from build123d import *

# Parameters (mm, degrees)
BOSS_EXTRUDE1_DEPTH    = 2
BOSS_EXTRUDE1_2_DEPTH  = 2
BOSS_EXTRUDE1_3_DEPTH  = 2
BOSS_EXTRUDE1_4_DEPTH  = 2
BOSS_EXTRUDE1_5_DEPTH  = 2
BOSS_EXTRUDE1_6_DEPTH  = 2
BOSS_EXTRUDE1_7_DEPTH  = 2
BOSS_EXTRUDE1_8_DEPTH  = 2
BOSS_EXTRUDE1_9_DEPTH  = 2
BOSS_EXTRUDE1_10_DEPTH = 2
SKETCH3_R              = 30
SKETCH3_R_2            = 16.5
BOSS_EXTRUDE2_DEPTH    = 2
SKETCH4_R              = 2.9
BOSS_EXTRUDE3_DEPTH    = 2
SKETCH6_R              = 5
BOSS_EXTRUDE4_DEPTH    = 1
SKETCH13_R             = 4.177329345
BOSS_EXTRUDE6_DEPTH    = 2
FILLET2_R              = 0.5
SKETCH14_R             = 3
CUT_EXTRUDE1_DEPTH     = 20


with BuildPart() as part:
    # Sketch2 → Boss-Extrude1 (new body)
    with BuildSketch(Plane.XY.offset(10)):
        with BuildLine():
            Line((8.357492916, 13.704694326), (1.290071734, 3.973134201))
            Line((1.290071734, 3.973134201), (1.290510646, 1.776982243))
            Line((1.290510646, 1.776982243), (3.379039645, 2.45604795))
            Line((3.379039645, 2.45604795), (10.446460828, 12.187608075))
            ThreePointArc((10.446460828, 12.187608075), (10.160519997, 13.990635156), (8.357492916, 13.704694326))
        make_face()
    extrude(amount=BOSS_EXTRUDE1_DEPTH)


with BuildPart() as body_2:
    # Sketch2 → Boss-Extrude1 2 (new body)
    with BuildSketch(Plane.XY.offset(10)):
        with BuildLine():
            Line((1.290071734, 3.973134201), (1.287668054, 16.000257666))
            ThreePointArc((1.287668054, 16.000257666), (-0.003455665, 17.290865413), (-1.294063412, 15.999741695))
            Line((-1.294063412, 15.999741695), (-1.291659732, 3.972618229))
            Line((-1.291659732, 3.972618229), (-0.000438912, 2.196151958))
            Line((-0.000438912, 2.196151958), (1.290071734, 3.973134201))
        make_face()
    extrude(amount=BOSS_EXTRUDE1_2_DEPTH)


with BuildPart() as body_3:
    # Sketch2 → Boss-Extrude1 3 (new body)
    with BuildSketch(Plane.XY.offset(10)):
        with BuildLine():
            Line((-1.29122082, 1.776466271), (-1.291659732, 3.972618229))
            Line((-1.291659732, 3.972618229), (-8.362970151, 13.701352658))
            ThreePointArc((-8.362970151, 13.701352658), (-10.166111381, 13.986572778), (-10.451331501, 12.183431547))
            Line((-10.451331501, 12.183431547), (-3.380021082, 2.454697118))
            Line((-3.380021082, 2.454697118), (-1.29122082, 1.776466271))
        make_face()
    extrude(amount=BOSS_EXTRUDE1_3_DEPTH)


with BuildPart() as body_4:
    # Sketch2 → Boss-Extrude1 4 (new body)
    with BuildSketch(Plane.XY.offset(10)):
        with BuildLine():
            Line((-2.088800262, 0.678230847), (-3.380021082, 2.454697118))
            Line((-3.380021082, 2.454697118), (-14.819238004, 6.168996626))
            ThreePointArc((-14.819238004, 6.168996626), (-16.445658083, 5.339884727), (-15.616546184, 3.713464648))
            Line((-15.616546184, 3.713464648), (-4.177329262, -0.00083486))
            Line((-4.177329262, -0.00083486), (-2.088800262, 0.678230847))
        make_face()
    extrude(amount=BOSS_EXTRUDE1_4_DEPTH)


with BuildPart() as body_5:
    # Sketch2 → Boss-Extrude1 5 (new body)
    with BuildSketch(Plane.XY.offset(10)):
        with BuildLine():
            Line((-2.088529, -0.679065707), (-4.177329262, -0.00083486))
            Line((-4.177329262, -0.00083486), (-15.615060628, -3.71970644))
            ThreePointArc((-15.615060628, -3.71970644), (-16.443522365, -5.346457793), (-14.816771011, -6.17491953))
            Line((-14.816771011, -6.17491953), (-3.379039645, -2.45604795))
            Line((-3.379039645, -2.45604795), (-2.088529, -0.679065707))
        make_face()
    extrude(amount=BOSS_EXTRUDE1_5_DEPTH)


with BuildPart() as body_6:
    # Sketch2 → Boss-Extrude1 6 (new body)
    with BuildSketch(Plane.XY.offset(10)):
        with BuildLine():
            Line((-1.290510646, -1.776982243), (-3.379039645, -2.45604795))
            Line((-3.379039645, -2.45604795), (-10.446460828, -12.187608075))
            ThreePointArc((-10.446460828, -12.187608075), (-10.160519997, -13.990635156), (-8.357492916, -13.704694326))
            Line((-8.357492916, -13.704694326), (-1.290071734, -3.973134201))
            Line((-1.290071734, -3.973134201), (-1.290510646, -1.776982243))
        make_face()
    extrude(amount=BOSS_EXTRUDE1_6_DEPTH)


with BuildPart() as body_7:
    # Sketch2 → Boss-Extrude1 7 (new body)
    with BuildSketch(Plane.XY.offset(10)):
        with BuildLine():
            Line((1.294063412, -15.999741695), (1.291659732, -3.972618229))
            Line((1.291659732, -3.972618229), (0.000438912, -2.196151958))
            Line((0.000438912, -2.196151958), (-1.290071734, -3.973134201))
            Line((-1.290071734, -3.973134201), (-1.287668054, -16.000257666))
            ThreePointArc((-1.287668054, -16.000257666), (0.003455665, -17.290865413), (1.294063412, -15.999741695))
        make_face()
    extrude(amount=BOSS_EXTRUDE1_7_DEPTH)


with BuildPart() as body_8:
    # Sketch2 → Boss-Extrude1 8 (new body)
    with BuildSketch(Plane.XY.offset(10)):
        with BuildLine():
            Line((10.451331501, -12.183431547), (3.380021082, -2.454697118))
            Line((3.380021082, -2.454697118), (1.29122082, -1.776466271))
            Line((1.29122082, -1.776466271), (1.291659732, -3.972618229))
            Line((1.291659732, -3.972618229), (8.362970151, -13.701352658))
            ThreePointArc((8.362970151, -13.701352658), (10.166111381, -13.986572778), (10.451331501, -12.183431547))
        make_face()
    extrude(amount=BOSS_EXTRUDE1_8_DEPTH)


with BuildPart() as body_9:
    # Sketch2 → Boss-Extrude1 9 (new body)
    with BuildSketch(Plane.XY.offset(10)):
        with BuildLine():
            Line((15.616546184, -3.713464648), (4.177329262, 0.00083486))
            Line((4.177329262, 0.00083486), (2.088800262, -0.678230847))
            Line((2.088800262, -0.678230847), (3.380021082, -2.454697118))
            Line((3.380021082, -2.454697118), (14.819238004, -6.168996626))
            ThreePointArc((14.819238004, -6.168996626), (16.445658083, -5.339884727), (15.616546184, -3.713464648))
        make_face()
    extrude(amount=BOSS_EXTRUDE1_9_DEPTH)


with BuildPart() as body_10:
    # Sketch2 → Boss-Extrude1 10 (new body)
    with BuildSketch(Plane.XY.offset(10)):
        with BuildLine():
            Line((14.816771011, 6.17491953), (3.379039645, 2.45604795))
            Line((3.379039645, 2.45604795), (2.088529, 0.679065707))
            Line((2.088529, 0.679065707), (4.177329262, 0.00083486))
            Line((4.177329262, 0.00083486), (15.615060628, 3.71970644))
            ThreePointArc((15.615060628, 3.71970644), (16.443522365, 5.346457793), (14.816771011, 6.17491953))
        make_face()
    extrude(amount=BOSS_EXTRUDE1_10_DEPTH)


with BuildPart() as body_11:
    # Sketch3 → Boss-Extrude2 (new body)
    with BuildSketch(Plane.XY.offset(12)):
        Circle(SKETCH3_R)
        Circle(SKETCH3_R_2, mode=Mode.SUBTRACT)
    extrude(amount=-BOSS_EXTRUDE2_DEPTH)

    # Sketch4 → Boss-Extrude3 (add)
    with BuildSketch(Plane.XY.offset(12)):
        with Locations((0, 25)):
            Circle(SKETCH4_R)
        with Locations((21.650635095, -12.5)):
            Circle(SKETCH4_R)
        with Locations((-21.650635095, -12.5)):
            Circle(SKETCH4_R)
    extrude(amount=BOSS_EXTRUDE3_DEPTH)

    # Sketch6 → Boss-Extrude4 (add)
    with BuildSketch(Plane(origin=(0, 0, 11), x_dir=(-1, 0, 0), z_dir=(0, 0, -1))):
        with Locations((0, 30)):
            Circle(SKETCH6_R)
        with Locations((25.980762114, -15)):
            Circle(SKETCH6_R)
        with Locations((-25.980762114, -15)):
            Circle(SKETCH6_R)
    extrude(amount=-BOSS_EXTRUDE4_DEPTH)


    add(part.part)  # Boss-Extrude6 merges part

    add(body_3.part)  # Boss-Extrude6 merges body 3

    add(body_5.part)  # Boss-Extrude6 merges body 5

    add(body_7.part)  # Boss-Extrude6 merges body 7

    add(body_9.part)  # Boss-Extrude6 merges body 9

    add(body_2.part)  # Boss-Extrude6 merges body 2

    add(body_4.part)  # Boss-Extrude6 merges body 4

    add(body_6.part)  # Boss-Extrude6 merges body 6

    add(body_8.part)  # Boss-Extrude6 merges body 8

    add(body_10.part)  # Boss-Extrude6 merges body 10
    # Sketch13 → Boss-Extrude6 (add)
    with BuildSketch(Plane(origin=(0, 0, 10), x_dir=(-1, 0, 0), z_dir=(0, 0, -1))):
        Circle(SKETCH13_R)
    extrude(amount=-BOSS_EXTRUDE6_DEPTH)

    # Fillet2
    fillet2_edges = [body_11.edges().sort_by_distance(p)[0] for p in [
        (-1.290071734, -3.973134201, 11),
        (1.291659732, -3.972618229, 11),
        (3.380021082, -2.454697118, 11),
        (4.177329262, 0.00083486, 11),
        (3.379039645, 2.45604795, 11),
        (1.290071734, 3.973134201, 11),
        (-1.291659732, 3.972618229, 11),
        (-3.380021082, 2.454697118, 11),
        (-4.177329262, -0.00083486, 11),
        (-3.379039645, -2.45604795, 11),
    ]]
    fillet(fillet2_edges, radius=FILLET2_R)

    # Sketch14 → Cut-Extrude1 (cut)
    with BuildSketch(Plane(origin=(0, 0, 10), x_dir=(-1, 0, 0), z_dir=(0, 0, -1))):
        Circle(SKETCH14_R)
    extrude(amount=-CUT_EXTRUDE1_DEPTH, mode=Mode.SUBTRACT)


solid = body_11.part
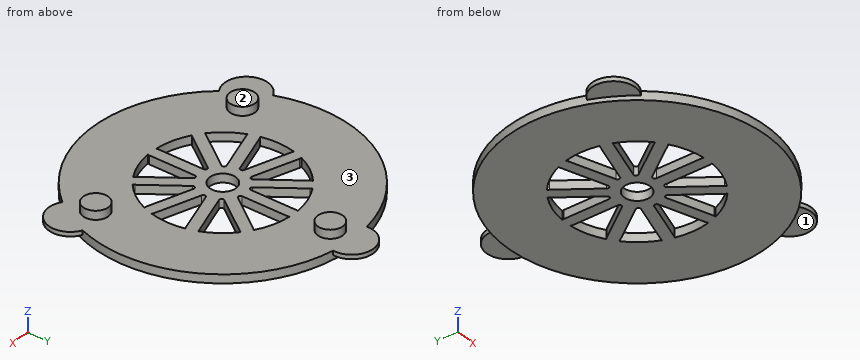
Geometry check sheet. Reference: the model listing, model coordinates, mm. Face numbers are marked on the shaded views. A direction names the side the tool comes from. Round coordinates to 2 decimals unless told otherwise and drop trailing zeros. Loops run counter-clockwise (first coordinate to the right, second up) from the corner with the lowest first, then second, coordinate; pieces in that order, holes last. Notation, with made-up numbers: (14, 55) -> (32, 55) arc R19 cw to (32, 78) -> close; hole circle Ø11 at (49, 63.25). An arc over 180 degrees is marked (long way). Answer as a JSON object with one key per item and string values. Group by question number.
Item 1: Cross-section at D-D, the plane x = -22. Record the cut outline in (y, z).
Item 2: Set-up check for the marked faces 1, 2 and 3: record each of +Z, -Z, +X, -X, +Y, -Y from which the full face is reachable in a straight line by a thin tool's end or side.
Item 3: Thickness scan on line 1 along Y through (x, z) = (0, 11.6); line 2 along Y through (x, z) = (0, 10.85); line 3 along Z through (x, y) = (-26, 12). Record the ranges inside material, lowest first.
Item 4: Cross-section at A-A, the plane x = -12.5. Record the cut outline in (y, z), plus the area to 3 significant figures.
Item 5: Cross-section at B-B, the plane z = 12.85. Record the cut outline in (x, y).
Item 6: Cross-section at C-C, the plane y = -7.5. Record the cut outline in (x, z), plus the area to 3 significant figures.
Item 7: Depth check by flat-ended pin: pin 1 Ø1.5 at (x, y) = (-2, -4) entering from +Z; pin 2 Ø2 at (y, z) = (-9, 11) entering from +X; pin 3 Ø1 at (y, z) = (12, 11) entering from -X; pin 4 Ø5 at (x, y) = (0, 0) entering from +Z. Enter the tip coordinate at first touch or a pass-through.
Determined:
{
 "1": {"outline": "(-20.4, 10) -> (20.4, 10) -> (20.4, 12) -> (-9.62, 12) -> (-9.62, 14) -> (-15.38, 14) -> (-15.38, 12) -> (-20.4, 12) -> close"},
 "2": {"face 1": "-Z, +X, -Y", "face 2": "+Z, +X, -X, +Y, -Y", "face 3": "+Z"},
 "3": {"line 1": "y = -30 to -3, 3 to 35", "line 2": "y = -30 to -3, 3 to 30", "line 3": "z = 10 to 12"},
 "4": {"outline": "(-27.27, 10) -> (-10.77, 10) -> (-10.77, 12) -> (-27.27, 12) -> close; (-5.42, 10) -> (-2.71, 10) -> (-2.71, 12) -> (-5.42, 12) -> close; (2.7, 10) -> (5.42, 10) -> (5.42, 12) -> (2.7, 12) -> close; (10.77, 10) -> (27.27, 10) -> (27.27, 12) -> (10.77, 12) -> close", "area": "76.9 mm²"},
 "5": {"outline": "circle Ø5.8 at (-21.65, -12.5); circle Ø5.8 at (0, 25); circle Ø5.8 at (21.65, -12.5)"},
 "6": {"outline": "(-29.05, 10) -> (-14.7, 10) -> (-14.7, 12) -> (-29.05, 12) -> close; (-7.04, 10) -> (-3.85, 10) -> (-3.85, 12) -> (-7.04, 12) -> close; (-1.29, 10) -> (1.29, 10) -> (1.29, 12) -> (-1.29, 12) -> close; (3.86, 10) -> (7.05, 10) -> (7.05, 12) -> (3.86, 12) -> close; (14.7, 10) -> (29.05, 10) -> (29.05, 12) -> (14.7, 12) -> close", "area": "75.3 mm²"},
 "7": {"pin 1": "stops at z = 12", "pin 2": "stops at x = 28.91", "pin 3": "stops at x = -27.71", "pin 4": "passes through"}
}
